```python
from build123d import *

# Parameters (mm, degrees)
F1_DEPTH = 2.54
F3_DEPTH = 2.541


with BuildPart() as f1:
    # F0 (on Front) → F1 (new body)
    with BuildSketch(Plane.XZ):
        with BuildLine():
            ThreePointArc((0, 3.81), (1.115923, 1.115923), (3.81, 0))
            Line((3.81, 0), (15.24, 0))
            ThreePointArc((15.24, 0), (17.934077, 1.115923), (19.05, 3.81))
            Line((19.05, 3.81), (19.05, 116.84))
            ThreePointArc((19.05, 116.84), (17.934077, 119.534077), (15.24, 120.65))
            Line((15.24, 120.65), (3.81, 120.65))
            ThreePointArc((3.81, 120.65), (1.115923, 119.534077), (0, 116.84))
            Line((0, 116.84), (0, 3.81))
        make_face()
    extrude(amount=F1_DEPTH)

    # F2 (on face) → F3 (cut, through all)
    with BuildSketch(Plane.XZ.offset(2.54)):
        with BuildLine():
            ThreePointArc((12.065, 110.49), (9.525, 113.03), (6.985, 110.49))
            Line((6.985, 110.49), (6.985, 85.725))
            ThreePointArc((6.985, 85.725), (9.525, 83.185), (12.065, 85.725))
            Line((12.065, 85.725), (12.065, 110.49))
        make_face()
        with BuildLine():
            ThreePointArc((6.985, 10.16), (9.525, 7.62), (12.065, 10.16))
            Line((12.065, 10.16), (12.065, 34.925))
            ThreePointArc((12.065, 34.925), (9.525, 37.465), (6.985, 34.925))
            Line((6.985, 34.925), (6.985, 10.16))
        make_face()
    extrude(amount=-F3_DEPTH, mode=Mode.SUBTRACT)


solid = f1.part
```
Check sheet for the modelled part. Datum: model origin and axes. Units: mm. A direction names the side the tool comes from. Coordinates: 2 decimals unless noted, no trailing zeros. Order: outer loops, then holes, each group sorted by start corner. A loop starts at its lowest first (then second) coordinate and runs counter-clockwise, first axis right, second up. Notation, with made-up numbers: (15.5, 73.5) -> (36.5, 73.5) arc R31 ccw to (36.5, 106.5) -> close; hole circle Ø6 at (-9.75, -20). An arc over 180 degrees is marked (long way). Write each question's results on one line, items separated by ' | '. Start each with the question number.
1) Depth check by flat-ended pin: pin 1 (1.5 mm diameter, centred on x = 15.5, y = -0.5, fed in from -Z). Enter the tip coordinate at first touch or a pass-through.
2) Section check C-C (x = 8.25). Enter the section's corners in (y, z), and give its area (3 significant figures).
3) Section check B-B (y = -1.85). Enter the section's corners in (x, z) (3 decimals).
4) Set-up check for faces 1 (the face through (9, -2.54, 61)), 2 (the face through (12.065, -1, 98)): record each of +Z, -Z, +X, -X, +Y, -Y from which the full face is reachable in a straight line by a thin tool's end or side.
5) Material ranges on line 1 along X through (y, z) = (-0.75, 106) (3 decimals); line 2 along Z through (x, y) = (8.25, -0.2), recorded low to high.
6) Section check A-A (z = 31). Enter the section's corners in (x, y) (3 decimals), and give its area (3 significant figures).
7) Draft check along Z on faces 3 (the face through (1.086, -1.252, 1.146)), 4 (the face through (6.985, -1, 23)), 5 (the face through (17.964, -1.252, 119.504)), 6 (the face through (12.065, -1, 22)). Enter one of: pulls with the +Z half, pulls with the -Z half, needs draft (parallel to the pull), parting line crosses it, or undercut.
Checked values:
1) pin 1: z = 0
2) outline: (-2.54, 0) -> (0, 0) -> (0, 7.96) -> (-2.54, 7.96) -> close; (-2.54, 37.12) -> (0, 37.12) -> (0, 83.53) -> (-2.54, 83.53) -> close; (-2.54, 112.69) -> (0, 112.69) -> (0, 120.65) -> (-2.54, 120.65) -> close | area: 158 mm²
3) outline: (0, 3.81) arc R3.81 ccw to (3.81, 0) -> (15.24, 0) arc R3.81 ccw to (19.05, 3.81) -> (19.05, 116.84) arc R3.81 ccw to (15.24, 120.65) -> (3.81, 120.65) arc R3.81 ccw to (0, 116.84) -> close; hole (6.985, 10.16) arc R2.54 ccw to (12.065, 10.16) -> (12.065, 34.925) arc R2.54 ccw to (6.985, 34.925) -> close; hole (6.985, 85.725) arc R2.54 ccw to (12.065, 85.725) -> (12.065, 110.49) arc R2.54 ccw to (6.985, 110.49) -> close
4) face 1: +Z, -Z, +X, -X, -Y | face 2: +Y, -Y
5) line 1: 0 to 6.985, 12.065 to 19.05 | line 2: 0 to 7.96, 37.12 to 83.53, 112.69 to 120.65
6) outline: (0, -2.54) -> (6.985, -2.54) -> (6.985, 0) -> (0, 0) -> close; (12.065, -2.54) -> (19.05, -2.54) -> (19.05, 0) -> (12.065, 0) -> close | area: 35.5 mm²
7) face 3: pulls with the -Z half | face 4: undercut | face 5: pulls with the +Z half | face 6: undercut
